Build history of the part. All positions in model axes, mm. A direction names the side the tool comes from. Round coordinates to 2 decimals unless told otherwise and drop trailing zeros. Loops run counter-clockwise (first coordinate to the right, second up) from the corner with the lowest first, then second, coordinate; pieces in that order, holes last. Notation, with made-up numbers: (13.5, 31.5) - (34.5, 31.5) arc R7 ccw to (34.5, 37.5) - close; hole circle Ø2 at (-1.75, 14). An arc over 180 degrees is marked (long way). Put each result on its own line as item: value. Start each with the question number.
from build123d import *

# Parameters (mm, degrees)
MASS_DEPTH                = 76.2
SKETCH17_W                = 63.5
SKETCH17_H                = 28.575
HOLLOW1_DEPTH             = 124.131068378
SKETCH19_W                = 50.8
SKETCH19_H                = 63.5
HOLLOW2_DEPTH             = 106.589636092
SKETCH20_R                = 9.652
HORIZ_BEARING_MOUNT_DEPTH = 105.389442115


with BuildPart() as part:
    # Sketch2 → Mass (new body)
    with BuildSketch(Plane.XY):
        with BuildLine():
            Line((0, 0), (60.325, 0))
            Line((60.325, 0), (60.325, 38.1))
            Line((60.325, 38.1), (0, 38.1))
            Line((0, 38.1), (-20.504465098, 26.524107549))
            ThreePointArc((-20.504465098, 26.524107549), (-27.282443066, 6.425609255), (-8.028287758, -2.472037758))
            Line((-8.028287758, -2.472037758), (0, 0))
        make_face()
    extrude(amount=MASS_DEPTH)

    # Sketch17 → Hollow1 (cut, through all)
    with BuildSketch(Plane(origin=(60.325, 0, 0), x_dir=(0, 0, -1), z_dir=(1, 0, 0))):
        with Locations((-38.1, 19.05)):
            Rectangle(SKETCH17_W, SKETCH17_H)
    extrude(amount=-HOLLOW1_DEPTH, mode=Mode.SUBTRACT)

    # Sketch19 → Hollow2 (cut, through all)
    with BuildSketch(Plane(origin=(0, 38.1, 0), x_dir=(1, 0, 0), z_dir=(0, 1, 0))):
        with Locations((-25.4, -38.1)):
            Rectangle(SKETCH19_W, SKETCH19_H)
    extrude(amount=-HOLLOW2_DEPTH, mode=Mode.SUBTRACT)

    # Sketch20 → Horiz. Bearing Mount (cut, through all)
    with BuildSketch(Plane.XY.offset(76.2)):
        with Locations((-12.7, 12.7)):
            Circle(SKETCH20_R)
    extrude(amount=-HORIZ_BEARING_MOUNT_DEPTH, mode=Mode.SUBTRACT)


solid = part.part
Item 1: Which spindle directions (+Z, -Z, +X, -X, +Y, -Y) get a long thin tool onto all of the face, cutting with end or side? Do faces 1 (the flat face through (25, 18, 0)), 2 (the flat face through (25, 18, 76.2)), 3 (the flat face through (31, 33.338, 39)), 4 (the flat face through (0, 36, 39)), 5 (the flat face through (30, 0, 38)). Say none if no direction does.
Item 2: Slice it at C-C (x = 54). Give the cut face in (y, z), plus the area to 3 significant figures.
Item 3: Drop flat-ended pins along their axis: pin 1 Ø20.5 at (x, y) = (24, 10) entering from -Z; pin 2 Ø12 at (y, z) = (15, 44.5) entering from +X; pin 3 Ø10 at (x, z) = (13, 35) entering from -Y; pin 4 Ø5 at (y, z) = (35, 37.5) entering from -X. Give the stop position or say it passes through.
Item 4: Slice it at A-A (z = 55). Give the cut face in (x, y) (1 decimal).
Item 5: Drill centre lines: probe 1 along Y at (x, z) = (27.5, 25.5); probe 2 along X at (y, z) = (13, 5) (3 decimals); probe 3 along Z at (x, y) = (-6.5, -0.5). Where is each one in solid material? Low to high. Write a range as [from, to].
Item 6: Slice it at B-B (y = 12.7). Give the cut face in (x, z) (3 decimals), plus the area to 3 significant figures.
Item 7: Two-plate mould, pull along Y, no slides. Class faces 6 (the flat face through (31, 4.763, 39)), 7 (the cylindrical face through (-7.51, 20.84, 73.07)), 8 (the flat face through (31, 38.1, 38)), 9 (the flat face through (-4.07, -1.253, 3.131)): pulls with the +Y half, pulls with the -Y half, needs draft (parallel to the pull), parting line crosses it, or undercut.
Item 8: Slice it at D-D (y = 25.5). Give the cut face in (x, z) (3 decimals).
Computed values:
1. face 1: -Z, +X, -X, +Y, -Y
1. face 2: +Z, +X, -X, +Y, -Y
1. face 3: +X, -X
1. face 4: -X, +Y, -Y
1. face 5: +Z, -Z, +X, -Y
2. outline: (0, 0) - (38.1, 0) - (38.1, 76.2) - (0, 76.2) - close; hole (4.76, 6.35) - (33.34, 6.35) - (33.34, 69.85) - (4.76, 69.85) - close
2. area: 1,090 mm^2
3. pin 1: stops at z = 0
3. pin 2: passes through
3. pin 3: stops at y = 0
3. pin 4: stops at x = 0
4. outline: (0, 0) - (60.3, 0) - (60.3, 4.8) - (0, 4.8) - close; (0, 33.3) - (60.3, 33.3) - (60.3, 38.1) - (0, 38.1) - close
5. probe 1: y = [0, 4.76], [33.34, 38.1]
5. probe 2: x = [-28.572, -22.347], [-3.053, 60.325]
5. probe 3: z = [0, 6.35], [69.85, 76.2]
6. outline: (-28.575, 0) - (-22.352, 0) - (-22.352, 6.35) - (-28.575, 6.35) - close; (-28.575, 69.85) - (-22.352, 69.85) - (-22.352, 76.2) - (-28.575, 76.2) - close; (-3.048, 0) - (60.325, 0) - (60.325, 6.35) - (-3.048, 6.35) - close; (-3.048, 69.85) - (60.325, 69.85) - (60.325, 76.2) - (-3.048, 76.2) - close
6. area: 884 mm^2
7. face 6: undercut
7. face 7: undercut
7. face 8: pulls with the +Y half
7. face 9: pulls with the -Y half
8. outline: (-22.09, 0) - (60.325, 0) - (60.325, 6.35) - (-22.09, 6.35) - close; (-22.09, 69.85) - (60.325, 69.85) - (60.325, 76.2) - (-22.09, 76.2) - close
